Could you check a few things on this model? Use its own coordinates, in mm. Face numbers are marked on the shaded views. A direction names the side the tool comes from. Round coordinates to 2 decimals unless told otherwise and drop trailing zeros. Loops run counter-clockwise (first coordinate to the right, second up) from the corner with the lowest first, then second, coordinate; pieces in that order, holes last. Notation, with made-up numbers: (88.25, 32.25) -> (124.25, 32.25) arc R22 ccw to (124.25, 69.25) -> close; hole circle Ø7 at (75, 75). An arc over 180 degrees is marked (long way). One line per item, written item: value.
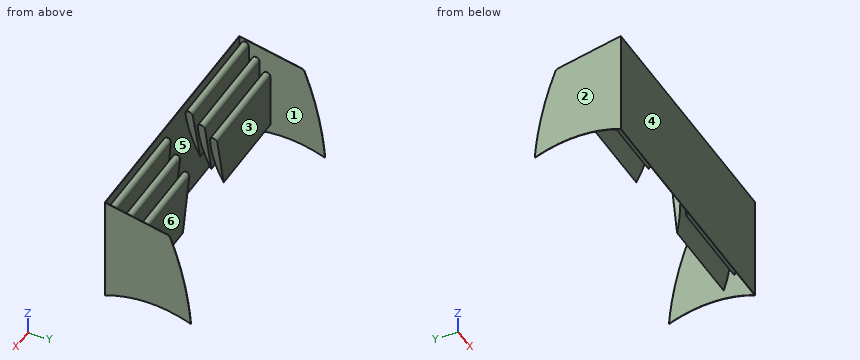
```python
from build123d import *

# Parameters (mm, degrees)
BOSS_EXTRUDE1_START      = 762
SKETCH1_W                = 635
SKETCH1_H                = 508
BOSS_EXTRUDE1_DEPTH      = 2.54
CUT_EXTRUDE1_DEPTH       = 1117.158775265
CUT_EXTRUDE1_DEPTH_BACK  = 1117.158775265
CUT_EXTRUDE2_DEPTH       = 1117.158775435
CUT_EXTRUDE2_DEPTH_BACK  = 1117.158775435
BOSS_EXTRUDE2_DEPTH      = 762
BOSS_EXTRUDE2_DEPTH_BACK = 764.54
SKETCH6_W                = 1529.0800025
SKETCH6_H                = 635
BOSS_EXTRUDE3_DEPTH      = 2.54
CUT_EXTRUDE3_DEPTH       = 182.122850144


with BuildPart() as part:
    # Sketch1 → Boss-Extrude1 (new body)
    with BuildSketch(Plane(origin=(0, 0, 0), x_dir=(0, 0, -1), z_dir=(1, 0, 0)).offset(BOSS_EXTRUDE1_START)):
        with Locations((317.5, 254)):
            Rectangle(SKETCH1_W, SKETCH1_H)
    extrude(amount=BOSS_EXTRUDE1_DEPTH)


with BuildPart() as body_2:
    # Mirror2: mirrored copy
    add(part.part.mirror(Plane(origin=(0, 0, 0), x_dir=(0, 0, 1), z_dir=(1, 0, 0))))


with BuildPart() as cut_extrude1_tool:
    # Sketch2 → Cut-Extrude1 (new, two sides: drawn at the far end of the back side and taken through both)
    with BuildSketch(Plane(origin=(0, 0, 0), x_dir=(0, 0, -1), z_dir=(1, 0, 0)).offset(-CUT_EXTRUDE1_DEPTH_BACK)):
        with BuildLine():
            Line((635, 508), (635, 0))
            add(Edge.make_bspline(
                [(635, 508), (535.978469305, 253.949693989), (635, 0)],
                knots=[0, 0, 0, 1, 1, 1], degree=2))
        make_face()
    extrude(amount=CUT_EXTRUDE1_DEPTH + CUT_EXTRUDE1_DEPTH_BACK)


with BuildPart() as part_1:
    add(part.part)

    # Cut-Extrude1: cut by cut_extrude1_tool
    add(cut_extrude1_tool.part, mode=Mode.SUBTRACT)


with BuildPart() as body_2_1:
    add(body_2.part)

    # Cut-Extrude1: cut by cut_extrude1_tool
    add(cut_extrude1_tool.part, mode=Mode.SUBTRACT)


with BuildPart() as cut_extrude2_tool:
    # Sketch3 → Cut-Extrude2 (new, two sides: drawn at the far end of the back side and taken through both)
    with BuildSketch(Plane(origin=(0, 0, 0), x_dir=(0, 0, -1), z_dir=(1, 0, 0)).offset(-CUT_EXTRUDE2_DEPTH_BACK)):
        with BuildLine():
            Line((0, 0), (78.126052631, 368.542434052))
            ThreePointArc((78.126052631, 368.542434052), (83.696209203, 379.813815366), (93.989588341, 387.033027713))
            add(Edge.make_bspline(
                [(635, 508), (448.701490757, 493.282812039), (268.257998273, 452.93411167), (93.989588341, 387.033027713)],
                knots=[0, 0, 0, 0, 0.975723085, 0.975723085, 0.975723085, 0.975723085], degree=3))
            Line((635, 508), (0, 508))
            Line((0, 508), (0, 0))
        make_face()
    extrude(amount=CUT_EXTRUDE2_DEPTH + CUT_EXTRUDE2_DEPTH_BACK)


with BuildPart() as part_2:
    add(part_1.part)

    # Cut-Extrude2: cut by cut_extrude2_tool
    add(cut_extrude2_tool.part, mode=Mode.SUBTRACT)



with BuildPart() as body_2_2:
    add(body_2_1.part)

    # Cut-Extrude2: cut by cut_extrude2_tool
    add(cut_extrude2_tool.part, mode=Mode.SUBTRACT)


with BuildPart() as part_3:
    add(part_2.part)

    add(body_2_2.part)  # Boss-Extrude2 merges body 2
    # Sketch4 → Boss-Extrude2 (add, two sides: drawn at the far end of the back side and taken through both)
    with BuildSketch(Plane(origin=(0, 0, 0), x_dir=(0, 0, -1), z_dir=(1, 0, 0)).offset(-BOSS_EXTRUDE2_DEPTH_BACK)):
        with BuildLine():
            Line((45.081165504, 57.724816481), (375.281165504, 64.574520115))
            add(Edge.make_bspline(
                [(375.281165504, 64.574520115), (213.984471731, 12.310346682), (45.081165504, 14.405048326)],
                knots=[0, 0, 0, 1, 1, 1], degree=2))
            ThreePointArc((45.081165504, 14.405048326), (23.421281427, 36.064932403), (45.081165504, 57.724816481))
        make_face()
        with BuildLine():
            Line((124.417436543, 121.193833312), (454.617436543, 121.193833312))
            add(Edge.make_bspline(
                [(454.617436543, 121.193833312), (292.934450552, 71.316103557), (124.417436543, 77.874065157)],
                knots=[0, 0, 0, 1, 1, 1], degree=2))
            ThreePointArc((124.417436543, 77.874065157), (102.757552466, 99.533949235), (124.417436543, 121.193833312))
        make_face()
        with BuildLine():
            Line((203.753707583, 184.662850144), (533.953707583, 184.662850144))
            add(Edge.make_bspline(
                [(203.753707583, 141.343081989), (373.054781607, 130.66856222), (533.953707583, 184.662850144)],
                knots=[0, 0, 0, 1, 1, 1], degree=2))
            ThreePointArc((203.753707583, 141.343081989), (182.093823506, 163.002966066), (203.753707583, 184.662850144))
        make_face()
    extrude(amount=BOSS_EXTRUDE2_DEPTH + BOSS_EXTRUDE2_DEPTH_BACK)

    # Sketch6 → Boss-Extrude3 (add)
    with BuildSketch(Plane(origin=(0, 0, 0), x_dir=(1, 0, 0), z_dir=(0, 1, 0))):
        with Locations((-1.25e-06, 317.5)):
            Rectangle(SKETCH6_W, SKETCH6_H)
    extrude(amount=BOSS_EXTRUDE3_DEPTH)

    # Sketch7 → Cut-Extrude3 (cut)
    with BuildSketch(Plane(origin=(0, 184.662850144, 0), x_dir=(1, 0, 0), z_dir=(0, 1, 0))):
        Polygon((-254, 635), (-114.3, 0), (114.3, 0), (254, 635), align=None)
    extrude(amount=-CUT_EXTRUDE3_DEPTH, mode=Mode.SUBTRACT)


solid = part_3.part
```
(1) Please list where these lines run through material, in increasing order: L1, parallel to X at y = 225, z = -169.5; L2, parallel to Y at x = 160, z = -44; L3, parallel to Y at x = 285, z = -178.
Results below:
L1: x = -764.54 to -762, 762 to 764.54
L2: y = 0 to 2.54, 14.43 to 57.7
L3: y = 0 to 2.54, 21.31 to 60.48, 77.22 to 121.19
(2) Imagine slicing it at A-A on x = 254. Give the number of separate pieces and of enclosed holes in the cut face, then the cut area to 3 significant figures.
Results below:
separate pieces: 4
enclosed holes: 0
area: 35,100 mm²
(3) On a 3-axis mill with a long thin cutter (end or side, diameter ignored), from which of +Z, -Z, +X, -X, +Y, -Y can I reach the whole of each face in a straight line? I mean the marked faces 4, 5 and 6. Say none if no direction works.
Results below:
face 4: +Z, -Z, +X, -X, -Y
face 5: +Z, -Z
face 6: +Z, -Z, +Y
(4) We'd pull the mould along Y, two halves only. Please class the marked faces 1, 2 and 3: +Y half, -Y half, draft (parallel to the pull), parting line (faces both ways), or undercut.
Results below:
face 1: undercut
face 2: draft
face 3: +Y half
(5) For pin 1 Ø1.5 at (x, z) = (401.5, -122) entering from +Y; pin 2 Ø12 at (x, z) = (-35.5, -322.5) entering from +Y, each with a flat end and sliding along its axis, tell me the tip position at first contact or that it passes through.
Results below:
pin 1: stops at y = 121.13
pin 2: stops at y = 2.54
(6) Imagine slicing it at B-B on x = 10. Write out the boundary of the cut face in (y, z), then the cut area to 3 significant figures.
Results below:
outline: (0, -635) -> (2.54, -635) -> (2.54, 0) -> (0, 0) -> close
area: 1,610 mm²
